Geometry: see drawing. Coordinates: mm, zero at the bounding-box minimum. A direction names the side the tool comes from. Give positions to 0.01 mm unless a question says otherwise; leave off trailing zeros. Order: outer loops, then holes, each group sorted by start corner. A loop starts at its lowest first (then second) coordinate and runs counter-clockwise, first axis right, second up. Notation, with made-up numbers: (77.25, 43.5) - (110.25, 43.5) arc R15 cw to (110.25, 53.5) - close; hole circle Ø8 at (15.25, 54.25). An arc over 180 degrees is marked (long way). Write item = value, one per line. Start each with the question number.
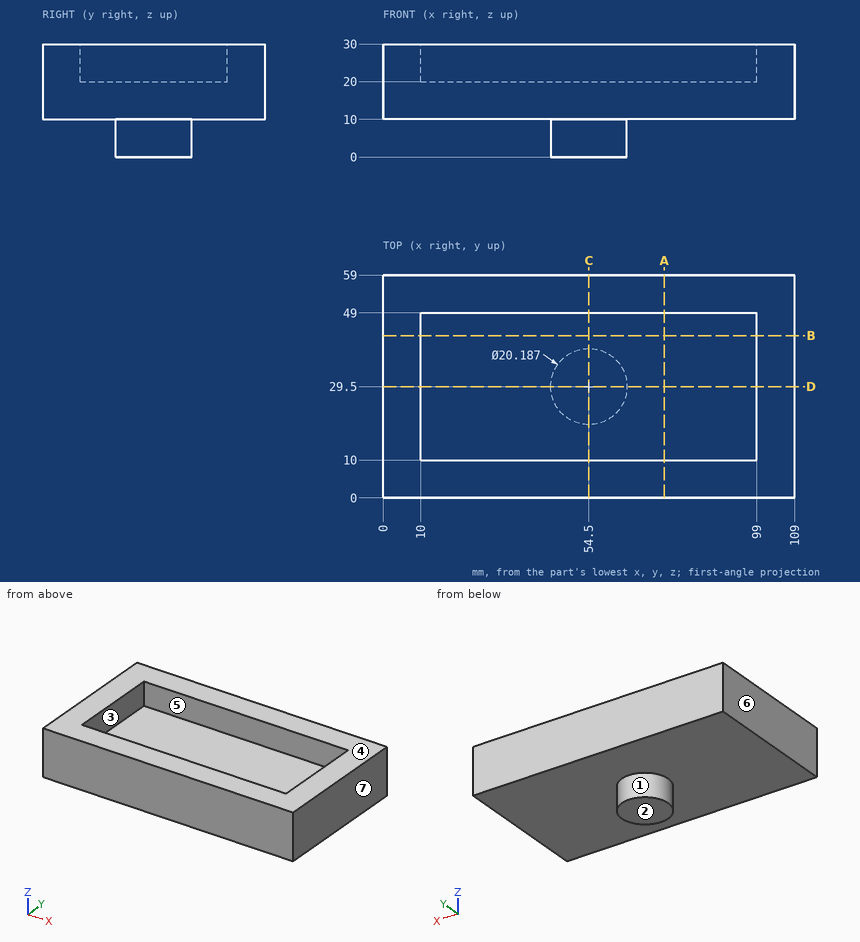
Q1. Pull-direction query (X, two-part tool) for the marked faces 4, 5, 6 and 7; classes: +X half, -X half, draft (parallel to the pull), parting line (faces both ways), or undercut.
Q2. Section A-A, the plane x = 74.5. Return the cut outline in (y, z).
Q3. Section D-D, the plane y = 29.5. Return the cut outline in (x, z), then the cut area to 3 significant figures.
Q4. Section C-C, the plane x = 54.5. Return the cut outline in (y, z), then the cut area to 3 significant figures.
Q5. Set-up query: the marked faces 1, 2 and 3. Return all of +Z, -Z, +X, -X, +Y, -Y with unobstructed straight access to the full face (end or side cutting, diameter ignored); none if empty.
Q6. Material intervals for line 1 along Y through (x, z) = (35.5, 25.75); line 2 along X through (y, z) = (34.5, 22); line 3 along Z through (x, y) = (48.5, 30.5), sorted ascending. Write a range as from..to.
Q7. Section B-B, the plane y = 43. Return the cut outline in (x, z).
Q8. Contact query for flat-ended pins moving along their axis: pin 1 (2 mm diameter, centred on x = 21, y = 28.5, fed in from -Z); pin 2 (5 mm diameter, centred on x = 48, z = 23, fed in from -Y); pin 3 (2 mm diameter, centred on x = 26.5, y = 29, fed in from +Z). Output: stop coordinate, or through.
The answers:
q1.face_4 = draft
q1.face_5 = undercut
q1.face_6 = -X half
q1.face_7 = +X half
q2.outline = (0, 10) - (59, 10) - (59, 30) - (49, 30) - (49, 20) - (10, 20) - (10, 30) - (0, 30) - close
q3.outline = (0, 10) - (44.41, 10) - (44.41, 0) - (64.59, 0) - (64.59, 10) - (109, 10) - (109, 30) - (99, 30) - (99, 20) - (10, 20) - (10, 30) - (0, 30) - close
q3.area = 1,490 mm²
q4.outline = (0, 10) - (19.41, 10) - (19.41, 0) - (39.59, 0) - (39.59, 10) - (59, 10) - (59, 30) - (49, 30) - (49, 20) - (10, 20) - (10, 30) - (0, 30) - close
q4.area = 992 mm²
q5.face_1 = -Z
q5.face_2 = -Z, +X, -X, +Y, -Y
q5.face_3 = +Z
q6.line_1 = 0..10, 49..59
q6.line_2 = 0..10, 99..109
q6.line_3 = 0..20
q7.outline = (0, 10) - (109, 10) - (109, 30) - (99, 30) - (99, 20) - (10, 20) - (10, 30) - (0, 30) - close
q8.pin_1 = 10
q8.pin_2 = 0
q8.pin_3 = 20
